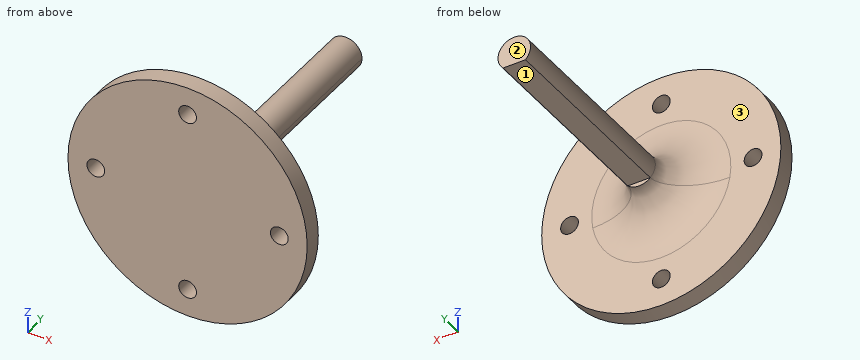
from build123d import *

# Parameters (mm, degrees)
SKETCH2_R           = 20.203446649
SKETCH2_R_2         = 1.5
SKETCH2_R_3         = 2.75
BOSS_EXTRUDE1_DEPTH = 3
BOSS_EXTRUDE2_DEPTH = 39.7
BOSS_EXTRUDE3_DEPTH = 6
FILLET1_SIZE        = 9
FILLET1_SIZE_2      = 6


with BuildPart() as part:
    # Sketch2 → Boss-Extrude1 (new body)
    # profile 1 of 5: a face of its own
    with BuildSketch(Plane(origin=(0, 0, 0), x_dir=(1, 0, 0), z_dir=(0, 1, 0))):
        with Locations(Location((0, 0, 0), (0, 0, 270))):
            Circle(SKETCH2_R)
        with Locations(Location((0, 15.5, 0), (0, 0, 270))):
            Circle(SKETCH2_R_2, mode=Mode.SUBTRACT)
        with Locations(Location((-15.5, 0, 0), (0, 0, 270))):
            Circle(SKETCH2_R_2, mode=Mode.SUBTRACT)
        with Locations(Location((0, -15.5, 0), (0, 0, 270))):
            Circle(SKETCH2_R_2, mode=Mode.SUBTRACT)
        with Locations(Location((15.5, 0, 0), (0, 0, 270))):
            Circle(SKETCH2_R_2, mode=Mode.SUBTRACT)
        Circle(SKETCH2_R_3, mode=Mode.SUBTRACT)
    # profile 2 of 5: a face of its own
    with BuildSketch(Plane(origin=(0, 0, 0), x_dir=(1, 0, 0), z_dir=(0, 1, 0))):
        with BuildLine():
            ThreePointArc((1.887458609, 2), (0, 2.75), (-1.887458609, 2))
            Line((-1.887458609, 2), (1.887458609, 2))
        make_face()
    # profile 3 of 5: a face of its own
    with BuildSketch(Plane(origin=(0, 0, 0), x_dir=(1, 0, 0), z_dir=(0, 1, 0))):
        with BuildLine():
            Line((1.887458609, 2), (-1.887458609, 2))
            ThreePointArc((-1.887458609, 2), (-1.089033706, -2.525174368), (2.75, 0))
            ThreePointArc((2.75, 0), (2.525174368, 1.089033706), (1.887458609, 2))
        make_face()
    # profile 4 of 5: a face of its own
    with BuildSketch(Plane(origin=(0, 0, 0), x_dir=(1, 0, 0), z_dir=(0, 1, 0))):
        with BuildLine():
            ThreePointArc((1.887458609, 2), (0, 2.75), (-1.887458609, 2))
            Line((-1.887458609, 2), (1.887458609, 2))
        make_face()
    # profile 5 of 5: a face of its own
    with BuildSketch(Plane(origin=(0, 0, 0), x_dir=(1, 0, 0), z_dir=(0, 1, 0))):
        with BuildLine():
            Line((1.887458609, 2), (-1.887458609, 2))
            ThreePointArc((-1.887458609, 2), (-1.089033706, -2.525174368), (2.75, 0))
            ThreePointArc((2.75, 0), (2.525174368, 1.089033706), (1.887458609, 2))
        make_face()
    extrude(amount=-BOSS_EXTRUDE1_DEPTH)

    # Sketch2<3> → Boss-Extrude2 (add)
    with BuildSketch(Plane(origin=(0, 0, 0), x_dir=(1, 0, 0), z_dir=(0, 1, 0))):
        with BuildLine():
            Line((1.887458609, 2), (-1.887458609, 2))
            ThreePointArc((-1.887458609, 2), (-1.089033706, -2.525174368), (2.75, 0))
            ThreePointArc((2.75, 0), (2.525174368, 1.089033706), (1.887458609, 2))
        make_face()
    extrude(amount=BOSS_EXTRUDE2_DEPTH)

    # Sketch2<4> → Boss-Extrude3 (add)
    with BuildSketch(Plane(origin=(0, 0, 0), x_dir=(1, 0, 0), z_dir=(0, 1, 0))):
        with BuildLine():
            ThreePointArc((1.887458609, 2), (0, 2.75), (-1.887458609, 2))
            Line((-1.887458609, 2), (1.887458609, 2))
        make_face()
        with BuildLine():
            Line((1.887458609, 2), (-1.887458609, 2))
            ThreePointArc((-1.887458609, 2), (-1.089033706, -2.525174368), (2.75, 0))
            ThreePointArc((2.75, 0), (2.525174368, 1.089033706), (1.887458609, 2))
        make_face()
    extrude(amount=BOSS_EXTRUDE3_DEPTH)

    # Fillet1
    # an asymmetric fillet: 9, 6 mm, written as the material it adds along each edge
    with BuildSketch(Plane(origin=(0, 0, 0), x_dir=(0.6863485850246134, 0, -0.7272727272727275), z_dir=(-0.7272727272727275, 0, -0.6863485850246134))) as fillet1_piece_1_section:
        with BuildLine():
            Bezier((2.75 + FILLET1_SIZE, 0), (2.75, 0), (2.75, -FILLET1_SIZE_2), weights=[1, 0.707106781, 1])
            Line((2.75, -FILLET1_SIZE_2), (2.75, 0))
            Line((2.75, 0), (2.75 + FILLET1_SIZE, 0))
        make_face()
    fillet1_piece_1 = revolve(axis=Axis((0, 0, 0), (0, -1, 0)), mode=Mode.PRIVATE)
    fillet1_piece_1 = split(fillet1_piece_1, bisect_by=Plane(origin=(2.77e-07, 0.848868766, -2), z_dir=(0, 0, -1)), keep=Keep.TOP, mode=Mode.PRIVATE)
    add(fillet1_piece_1)
    with BuildSketch(Plane(origin=(0, 0, 0), x_dir=(0.6863485850246134, 0, -0.7272727272727275), z_dir=(-0.7272727272727275, 0, -0.6863485850246134))) as fillet1_piece_2_section:
        with BuildLine():
            Bezier((2.75 + FILLET1_SIZE, 0), (2.75, 0), (2.75, -FILLET1_SIZE_2), weights=[1, 0.707106781, 1])
            Line((2.75, -FILLET1_SIZE_2), (2.75, 0))
            Line((2.75, 0), (2.75 + FILLET1_SIZE, 0))
        make_face()
    fillet1_piece_2 = revolve(axis=Axis((0, 0, 0), (0, -1, 0)), mode=Mode.PRIVATE)
    fillet1_piece_2 = split(fillet1_piece_2, bisect_by=Plane(origin=(-3.3e-08, 1.056267752, -2), z_dir=(0, 0, 1)), keep=Keep.TOP, mode=Mode.PRIVATE)
    add(fillet1_piece_2)


solid = part.part
Check sheet for the modelled part. Datum: model origin and axes. Units: mm. Face numbers are marked on the shaded views. A direction names the side the tool comes from. Coordinates: 2 decimals unless noted, no trailing zeros. Loops run counter-clockwise (first coordinate to the right, second up) from the corner with the lowest first, then second, coordinate; pieces in that order, holes last. Notation, with made-up numbers: (20.25, 64.25) -> (42.25, 64.25) arc R20 cw to (42.25, 77.25) -> close; hole circle Ø1 at (59, 37.25). An arc over 180 degrees is marked (long way). Answer in a Markdown table with one row per item.
1. Sectioned sample at A-A, the plane x = 15.5. Record the boundary of the cut face in (y, z), then the cut area to 3 significant figures.
Check values:
| item | result |
|---|---|
| outline | (-3, -12.96) -> (0, -12.96) -> (0, -1.5) -> (-3, -1.5) -> close; (-3, 1.5) -> (0, 1.5) -> (0, 12.96) -> (-3, 12.96) -> close |
| area | 68.8 mm2 |
2. Go/stop test with flat-tipped pins: pin 1 (1 mm diameter, centred on x = 1.5, y = 17, fed in from -Z); pin 2 (0.8 mm diameter, centred on x = 1, z = -2.5, fed in from +Y); pin 3 (1.5 mm diameter, centred on x = -0.5, z = 6.5, fed in from +Y). Record where each tip stops, or that it passes through.
Check values:
| item | result |
|---|---|
| pin 1 | stops at z = -2 |
| pin 2 | stops at y = 6 |
| pin 3 | stops at y = 1.52 |
3. Sectioned sample at D-D, the plane y = 20. Record the boundary of the cut face in (x, z).
Check values:
| item | result |
|---|---|
| outline | (-1.89, -2) -> (1.89, -2) arc R2.75 ccw (long way) to start |
4. Sectioned sample at C-C, the plane x = 0. Give the number of separate pieces and of enclosed holes in the cut face, then the cut area to 3 significant figures.
Check values:
| item | result |
|---|---|
| separate pieces | 3 |
| enclosed holes | 0 |
| area | 319 mm2 |
5. Sectioned sample at B-B, the plane z = 15.5. Record the boundary of the cut face in (x, y).
Check values:
| item | result |
|---|---|
| outline | (-12.96, -3) -> (-1.5, -3) -> (-1.5, 0) -> (-12.96, 0) -> close; (1.5, -3) -> (12.96, -3) -> (12.96, 0) -> (1.5, 0) -> close |
6. Access from +Z, -Z, +X, -X, +Y, -Y to the whole of each face (thin tool, end or side, straight path). Record for the marked faces 1, 2 and 3.
Check values:
| item | result |
|---|---|
| face 1 | -Z, +X, -X, +Y |
| face 2 | +Z, -Z, +X, -X, +Y |
| face 3 | +Y |
7. Material ranges on line 1 along X through (y, z) = (-2, 0); line 2 along Y through (x, z) = (7, -9); line 3 along X through (y, z) = (-1.8, 15.5), recorded low to high. Write a range as [from, to].
Check values:
| item | result |
|---|---|
| line 1 | x = [-20.2, -17], [-14, 14], [17, 20.2] |
| line 2 | y = [-3, 0] |
| line 3 | x = [-12.96, -1.5], [1.5, 12.96] |
